Drawing for the job (mm, zero at the part's lowest x, y, z). A direction names the side the tool comes from. Coordinates: 2 decimals unless noted, no trailing zeros. Write each loop counter-clockwise with the first axis right and the second up, starting at its lowest first coordinate (ties: lowest second). Pieces come first, ordered by that corner, then holes. Notation, with made-up numbers: M 87.5,-7.75 L 137.5,-7.75 A24 ccw 137.5,30.25 Z; hole C -11,57 d8. An arc over 180 degrees is marked long. Put each result on its own line as item: value. Start each with the question number.
Q1. Drill centre lines: line 1 along Z through (x, y) = (10.5, 5.75); line 2 along X through (y, z) = (6.5, 15.25); line 3 along Z through (x, y) = (23.75, 3.75). Where is each one in solid material? Low to high.
Q2. Which spindle directions (+Z, -Z, +X, -X, +Y, -Y) get a long thin tool onto all of the face, cutting with end or side? Do the marked faces 5, 6, 7 and 8. Say none if no direction does.
Q3. Drop flat-ended pins along their axis: pin 1 (1.4 mm diameter, centred on x = 10.5, y = 4, fed in from +Z); pin 2 (1.5 mm diameter, centred on y = 2.5, z = 13, fed in from -X); pin 3 (3 mm diameter, centred on x = 7, y = 2, fed in from +Z); pin 4 (8 mm diameter, centred on x = 14, z = 11.5, fed in from -Y). Give the stop position or say it passes through.
Q4. Cut at D-D (x = 9). Write the cut outline in (y, z).
Q5. Cut at B-B (x = 3.25). Write the cut outline in (y, z).
Q6. Pull direction X, two halves, no side cores. Call the marked faces 1, 2, 3 and 4: pulls with the +X half, pulls with the -X half, needs draft (parallel to the pull), parting line crosses it, or undercut.
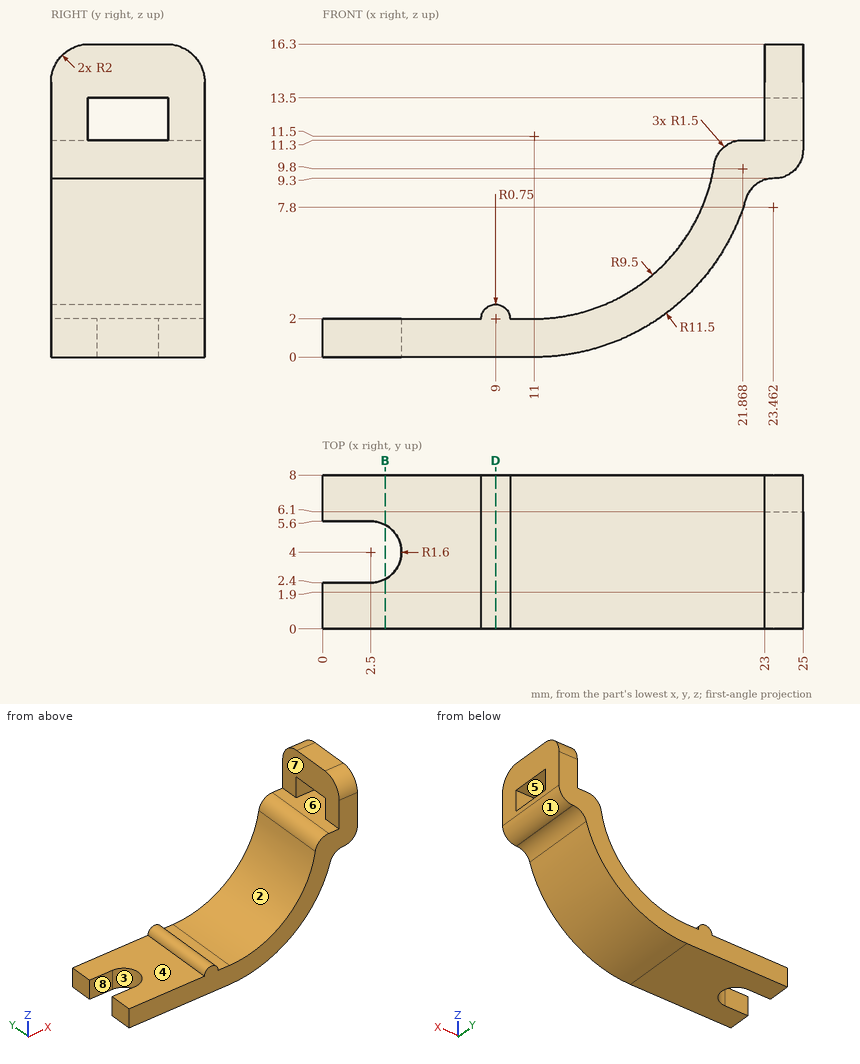
Computed values:
1. line 1: 0 to 2
1. line 2: 23 to 25
1. line 3: 9.32 to 11.3, 13.5 to 16.3
2. face 5: +X, -X
2. face 6: -X
2. face 7: +Z, -X, +Y, -Y
2. face 8: +Z, -Z, -X
3. pin 1: z = 2
3. pin 2: x = 23
3. pin 3: z = 2.56
3. pin 4: through
4. outline: M 0,0 L 8,0 L 8,2.75 L 0,2.75 Z
5. outline: M 0,0 L 2.59,0 L 2.59,2 L 0,2 Z; M 5.41,0 L 8,0 L 8,2 L 5.41,2 Z
6. face 1: pulls with the +X half
6. face 2: undercut
6. face 3: pulls with the -X half
6. face 4: needs draft
